from build123d import *

# Parameters (mm, degrees)
F0_W     = 157.5917825103
F0_H     = 105.6277751923
F1_DEPTH = 50.8
F2_W     = 55.120697245
F2_H     = 24.0394249558
F3_DEPTH = 25.4
F2_W_2   = 62.8910250962
F2_H_2   = 89.8443162441
F4_DEPTH = 25.4


with BuildPart() as f1:
    # F0 (on Front) → F1 (new body)
    with BuildSketch(Plane.XZ):
        with Locations((2.6710517704, 2.549637109)):
            Rectangle(F0_W, F0_H)
    extrude(amount=F1_DEPTH)

    # F2 (on face) → F3 (cut)
    with BuildSketch(Plane.XZ.offset(50.8)):
        with Locations((-48.5644908622, 43.3438122272)):
            Rectangle(F2_W, F2_H)
    extrude(amount=-F3_DEPTH, mode=Mode.SUBTRACT)

    # F2 (on face) → F4 (cut)
    with BuildSketch(Plane.XZ.offset(50.8)):
        with Locations((50.0214304775, 10.4413665831)):
            Rectangle(F2_W_2, F2_H_2)
    extrude(amount=-F4_DEPTH, mode=Mode.SUBTRACT)


solid = f1.part
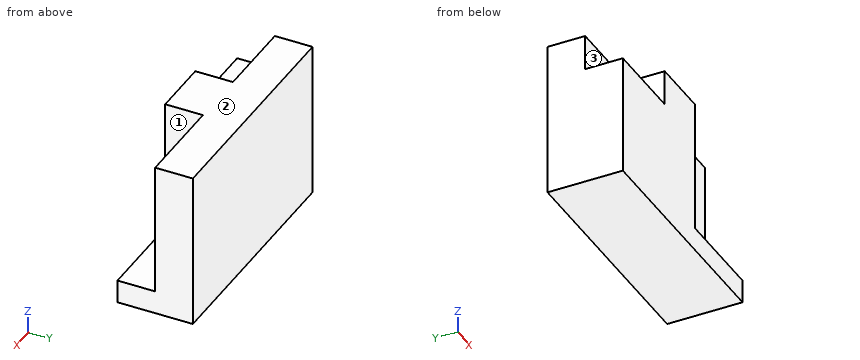
Design review of the part built by this model. Coordinates are the model's own, in mm. Face numbers are marked on the shaded views. A direction names the side the tool comes from. Coordinates: 2 decimals unless noted, no trailing zeros. Order: outer loops, then holes, each group sorted by start corner. A loop starts at its lowest first (then second) coordinate and runs counter-clockwise, first axis right, second up. Notation, with made-up numbers: M 57.25,-38.5 L 82.25,-38.5 A27 cw 82.25,-4.5 Z; hole C 34,24 d11. An arc over 180 degrees is marked long. Use a Markdown table: item, result.
(1) Add section B-B (z = 43.5). Give the boundary of the cut face in (x, y), then the cut area to 3 significant figures.
Worked answers:
| item | result |
|---|---|
| outline | M -76.12,-25.4 L -21,-25.4 L -21,-50.8 L 18.58,-50.8 L 18.58,-25.4 L 81.47,-25.4 L 81.47,0 L -76.12,0 Z |
| area | 5,010 mm2 |
(2) Add section D-D (z = 12). Give the boundary of the cut face in (x, y), then the cut area to 3 significant figures.
Worked answers:
| item | result |
|---|---|
| outline | M -76.12,-50.8 L 18.58,-50.8 L 18.58,-25.4 L 81.47,-25.4 L 81.47,0 L -76.12,0 Z |
| area | 6,410 mm2 |
(3) For P1, Ø7.5, axis at x = -60, y = -35.5, coming from the +Z side; P2, Ø1.5, axis at x = 25, y = -41.5, coming from the +Z side; P3, Ø7.5, axis at y = -35, z = 27, coming from the +X side, all flat-tipped, find the tip position at first contact; note any pin that passes through.
Worked answers:
| item | result |
|---|---|
| P1 | stops at z = 31.32 |
| P2 | stops at z = -34.48 |
| P3 | stops at x = 18.58 |
(4) For the marked faces 1, 2 and 3, list the 3-axis set-ups (+Z, -Z, +X, -X, +Y, -Y) from which the entire face can be reached by the end or side of a thin tool; tool diameter is ignored.
Worked answers:
| item | result |
|---|---|
| face 1 | +Z, +X, -Y |
| face 2 | +Z, +X, -X, +Y, -Y |
| face 3 | +Z, -X, -Y |
(5) Add section A-A (y = -29). Give the boundary of the cut face in (x, z), then the cut area to 3 significant figures.
Worked answers:
| item | result |
|---|---|
| outline | M -76.12,-50.26 L 81.47,-50.26 L 81.47,-34.48 L 18.58,-34.48 L 18.58,55.36 L -21,55.36 L -21,31.32 L -76.12,31.32 Z |
| area | 9,670 mm2 |
(6) Add section C-C (x = -59.5). Give the boundary of the cut face in (y, z).
Worked answers:
| item | result |
|---|---|
| outline | M -50.8,-50.26 L 0,-50.26 L 0,55.36 L -25.4,55.36 L -25.4,31.32 L -50.8,31.32 Z |
(7) Wall thickness on probe 1 along Y at (x, z) = (56, 31); probe 2 along X at (y, z) = (-33, -31); probe 3 along Z at (x, y) = (-68.5, -33): over which ranges is each line inside the solid? List them lowest first.
Worked answers:
| item | result |
|---|---|
| probe 1 | y = -25.4 to 0 |
| probe 2 | x = -76.12 to 18.58 |
| probe 3 | z = -50.26 to 31.32 |
